Autodesk Inventor part; units mm, degrees
ref_plane "YZ Plane" through (0, 0, 0) normal (1, 0, 0) x (0, 1, 0)
ref_plane "XZ Plane" through (0, 0, 0) normal (0, 1, 0) x (-1, 0, 0)
ref_plane "XY Plane" through (0, 0, 0) normal (0, 0, 1) x (1, 0, 0)
sketch "Sketch1" plane through (0, 0, 0) normal (0, 1, 0) x (-1, 0, 0)
  circle A0 centre (0, 0) radius 5.25
  line L0 (0, 0) -> (0, 23.5)
  circle A1 centre (0, 23.5) radius 10.5
  line L1 (0, 23.5) -> (14, 23.5)
  line L2 (14, 23.5) -> (14, 36.5)
  line L3 (14, 36.5) -> (-14, 36.5)
  line L4 (-14, 36.5) -> (-14, -18.25)
  line L5 (-14, -18.25) -> (-16.5, -18.25)
  line L6 (-16.5, -18.25) -> (-16.5, -38.5)
  line L7 (14, 23.5) -> (14, -38.5)
  spline S0 degree 4 poles (14, -38.5) (9.1992, -54.9126) (-5.1458, -16.9331) (-9.6244, -54.3444) (-16.5, -38.5) knots 0 0 0 0 0 1 1 1 1 1
  point P0 (7, -41.75)
  point P1 (-3, -38.5)
  point P2 (-10.5, -41.75)
  dimension "d0" = 10.5
  dimension "d2" = 23.5
  dimension "d3" = 21
  dimension "d4" = 14
  dimension "d5" = 13
  dimension "d6" = 28
  dimension "d7" = 54.75
  dimension "d8" = 2.5
  dimension "d9" = 20.25
  dimension "d10" = 62
extrude "Extrusion1" add sketch "Sketch1" along normal blind 2
properties part number "Tira"
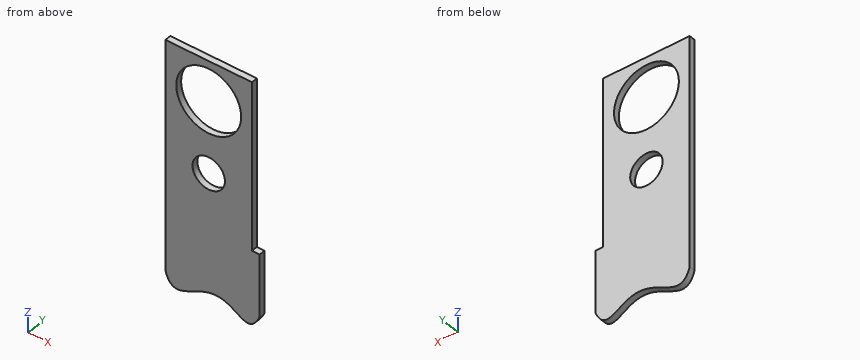
Input: part model. Units: mm. Frame: model coordinates. Give positions to 0.01 mm unless a question says otherwise; leave off trailing zeros. Loops run counter-clockwise (first coordinate to the right, second up) from the corner with the lowest first, then second, coordinate; pieces in that order, holes last. Notation, with made-up numbers: (-31.5, -16) - (5.5, -16) arc R15 ccw to (5.5, 13) - close; hole circle Ø2 at (-15, 9.25). An arc over 180 degrees is marked (long way). Use CSV: the item, a comma, the result in double quotes. Start each with the question number.
Item 1: Section D-D on z = -11.5. Return loops of the section in (x, y), then the cut area to 3 significant figures.
Item 2: Section B-B on z = 0. Return loops of the section in (x, y), then the cut area to 3 significant figures.
Item 3: Section C-C on y = 1.65. State how many separate pieces and enclosed holes the cut face has, then the cut area to 3 significant figures.
Item 4: Line query: line 1 (Z direction, x = 0, y = 1.5); line 2 (Z direction, x = -1.5, y = 1.05); line 3 (X direction, y = 1, z = -1.5). Output: solid intervals per line, ascending.
Item 5: Contact query for flat-ended pins moving along their axis: P1, Ø4, axis at x = 4.5, z = 2.5, coming from the +Y side; P2, Ø0.6, axis at x = 15.5, y = 0.5, coming from the +Z side; P3, Ø1, axis at x = 13, y = 1, coming from the -Z side. Output: stop coordinate, or through.
Item 6: Section A-A on z = 23.5. Return loops of the section in (x, y), then the cut area to 3 significant figures.
Ans:
1,outline,"(-14, 0) - (14, 0) - (14, 2) - (-14, 2) - close"
1,area,"56.0 mm2"
2,outline,"(-14, 0) - (-5.25, 0) - (-5.25, 2) - (-14, 2) - close; (5.25, 0) - (14, 0) - (14, 2) - (5.25, 2) - close"
2,area,"35.0 mm2"
3,separate pieces,"1"
3,enclosed holes,"2"
3,area,"1,780 mm2"
4,line 1,"z = -38.77 to -5.25, 5.25 to 13, 34 to 36.5"
4,line 2,"z = -39.22 to -5.03, 5.03 to 13.11, 33.89 to 36.5"
4,line 3,"x = -14 to -5.03, 5.03 to 14"
5,P1,"stops at y = 2"
5,P2,"stops at z = -18.25"
5,P3,"stops at z = -42.43"
6,outline,"(-14, 0) - (-10.5, 0) - (-10.5, 2) - (-14, 2) - close; (10.5, 0) - (14, 0) - (14, 2) - (10.5, 2) - close"
6,area,"14.0 mm2"
